Could you check a few things on this drawing? It's one solid part, dimensions in mm from its lowest x, y, z. A direction names the side the tool comes from. Coordinates: 2 decimals unless noted, no trailing zeros. Write each loop counter-clockwise with the first axis right and the second up, starting at its lowest first coordinate (ties: lowest second). Pieces come first, ordered by that corner, then holes. Notation, with made-up numbers: (-27, 71) - (-4, 71) arc R24 cw to (-4, 82) - close; hole circle Ø5 at (-13, 79). An arc over 180 degrees is marked (long way). Answer as a JSON object with one key per item and string values. Group by question number.
1) We'd pull the mould along Z, two halves only. Please class the marked faces 1, 2, 3 and 4: released by +Z, released by -Z, zero draft, split by the parting line, or undercut.
2) On a 3-axis mill with a long thin cutter (end or side, diameter ignored), from which of +Z, -Z, +X, -X, +Y, -Y can I reach the whole of each face in a straight line? I mean the marked faces 5, 6 and 7. Say none if no direction works.
3) Please list where these lines run through material, in increasing order: line 1 along X through (y, z) = (5.5, 2); line 2 along Z through (x, y) = (18.5, 6.25); line 3 along X through (y, z) = (0.75, 1.25).
4) If we section it at A-A (x = 13.5): Write out the boundary of the cut face in (y, z).
5) If we section it at C-C (z = 2): Write out the boundary of the cut face in (x, y), plus the area to 3 significant figures.
6) If we section it at D-D (x = 22.5): Write out the boundary of the cut face in (y, z).
7) Will these pins go through, and if not, where does the flat tip stop? pin 1 Ø1 at (x, y) = (21.5, 5.5) entering from +Z; pin 2 Ø2.5 at (x, y) = (4.5, 3.5) entering from -Z.
8) If we section it at B-B (y = 2): Write out the boundary of the cut face in (x, z).
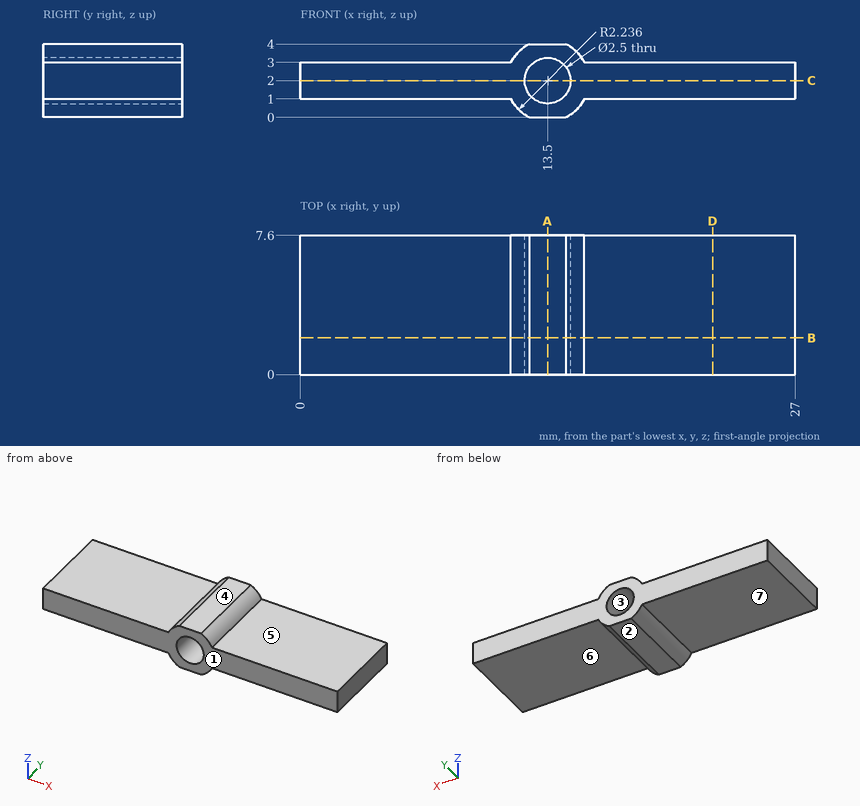
Here are the results:
{
 "1": {"face 1": "zero draft", "face 2": "released by -Z", "face 3": "undercut", "face 4": "released by +Z"},
 "2": {"face 5": "+Z, +X, +Y, -Y", "face 6": "-Z, +X, +Y, -Y", "face 7": "-Z, -X, +Y, -Y"},
 "3": {"line 1": "x = 0 to 12.25, 14.75 to 27", "line 2": "z = 1 to 3", "line 3": "x = 0 to 12.5, 14.5 to 27"},
 "4": {"outline": "(0, 0) - (7.6, 0) - (7.6, 0.75) - (0, 0.75) - close; (0, 3.25) - (7.6, 3.25) - (7.6, 4) - (0, 4) - close"},
 "5": {"outline": "(0, 0) - (12.25, 0) - (12.25, 7.6) - (0, 7.6) - close; (14.75, 0) - (27, 0) - (27, 7.6) - (14.75, 7.6) - close", "area": "186 mm²"},
 "6": {"outline": "(0, 1) - (7.6, 1) - (7.6, 3) - (0, 3) - close"},
 "7": {"pin 1": "stops at z = 3", "pin 2": "stops at z = 1"},
 "8": {"outline": "(0, 1) - (11.5, 1) arc R2.24 ccw to (12.5, 0) - (14.5, 0) arc R2.24 ccw to (15.5, 1) - (27, 1) - (27, 3) - (15.5, 3) arc R2.24 ccw to (14.5, 4) - (12.5, 4) arc R2.24 ccw to (11.5, 3) - (0, 3) - close; hole circle Ø2.5 at (13.5, 2)"}
}
